The model under review builds one solid part; all positions refer to its coordinate system, in mm. Coordinates: 2 decimals unless noted, no trailing zeros. Write each question's results on one line, items separated by ' | '.
from build123d import *

# Parameters (mm, degrees)
EXTRUDE1_DEPTH = 406.4


with BuildPart() as part:
    # Sketch1 → Extrude1 (new body)
    with BuildSketch(Plane.XY):
        with BuildLine():
            Line((8.3439, -10.4902), (6.225100202, -10.4902))
            ThreePointArc((6.225100202, -10.4902), (5.286438597, -9.863006367), (5.506679712, -8.75577951))
            Line((5.506679712, -8.75577951), (8.81535611, -5.447103113))
            ThreePointArc((8.81535611, -5.447103113), (9.845400242, -4.758849627), (11.06042014, -4.517167143))
            Line((11.06042014, -4.517167143), (14.33957986, -4.517167143))
            ThreePointArc((14.33957986, -4.517167143), (15.554599758, -4.758849627), (16.58464389, -5.447103113))
            Line((16.58464389, -5.447103113), (19.893320288, -8.75577951))
            ThreePointArc((19.893320288, -8.75577951), (20.113561403, -9.863006367), (19.174899798, -10.4902))
            Line((19.174899798, -10.4902), (17.0561, -10.4902))
            ThreePointArc((17.0561, -10.4902), (15.9512, -11.5951), (17.0561, -12.7))
            Line((17.0561, -12.7), (23.2918, -12.7))
            ThreePointArc((23.2918, -12.7), (24.782522516, -12.082522516), (25.4, -10.5918))
            Line((25.4, -10.5918), (25.4, -4.3561))
            ThreePointArc((25.4, -4.3561), (24.2951, -3.2512), (23.1902, -4.3561))
            Line((23.1902, -4.3561), (23.1902, -6.474899798))
            ThreePointArc((23.1902, -6.474899798), (22.563006367, -7.413561403), (21.45577951, -7.193320288))
            Line((21.45577951, -7.193320288), (18.147103113, -3.88464389))
            ThreePointArc((18.147103113, -3.88464389), (17.458849627, -2.854599758), (17.217167143, -1.63957986))
            Line((17.217167143, -1.63957986), (17.217167143, 1.63957986))
            ThreePointArc((17.217167143, 1.63957986), (17.458849627, 2.854599758), (18.147103113, 3.88464389))
            Line((18.147103113, 3.88464389), (21.45577951, 7.193320288))
            ThreePointArc((21.45577951, 7.193320288), (22.563006367, 7.413561403), (23.1902, 6.474899798))
            Line((23.1902, 6.474899798), (23.1902, 4.3561))
            ThreePointArc((23.1902, 4.3561), (24.2951, 3.2512), (25.4, 4.3561))
            Line((25.4, 4.3561), (25.4, 10.5918))
            ThreePointArc((25.4, 10.5918), (24.782522516, 12.082522516), (23.2918, 12.7))
            Line((23.2918, 12.7), (17.0561, 12.7))
            ThreePointArc((17.0561, 12.7), (15.9512, 11.5951), (17.0561, 10.4902))
            Line((17.0561, 10.4902), (19.174899798, 10.4902))
            ThreePointArc((19.174899798, 10.4902), (20.113561403, 9.863006367), (19.893320288, 8.75577951))
            Line((19.893320288, 8.75577951), (16.58464389, 5.447103113))
            ThreePointArc((16.58464389, 5.447103113), (15.554599758, 4.758849627), (14.33957986, 4.517167143))
            Line((14.33957986, 4.517167143), (11.06042014, 4.517167143))
            ThreePointArc((11.06042014, 4.517167143), (9.845400242, 4.758849627), (8.81535611, 5.447103113))
            Line((8.81535611, 5.447103113), (5.506679712, 8.75577951))
            ThreePointArc((5.506679712, 8.75577951), (5.286438597, 9.863006367), (6.225100202, 10.4902))
            Line((6.225100202, 10.4902), (8.3439, 10.4902))
            ThreePointArc((8.3439, 10.4902), (9.4488, 11.5951), (8.3439, 12.7))
            Line((8.3439, 12.7), (-8.3439, 12.7))
            ThreePointArc((-8.3439, 12.7), (-9.4488, 11.5951), (-8.3439, 10.4902))
            Line((-8.3439, 10.4902), (-6.225100202, 10.4902))
            ThreePointArc((-6.225100202, 10.4902), (-5.286438597, 9.863006367), (-5.506679712, 8.75577951))
            Line((-5.506679712, 8.75577951), (-8.81535611, 5.447103113))
            ThreePointArc((-8.81535611, 5.447103113), (-9.845400242, 4.758849627), (-11.06042014, 4.517167143))
            Line((-11.06042014, 4.517167143), (-14.33957986, 4.517167143))
            ThreePointArc((-14.33957986, 4.517167143), (-15.554599758, 4.758849627), (-16.58464389, 5.447103113))
            Line((-16.58464389, 5.447103113), (-19.893320288, 8.75577951))
            ThreePointArc((-19.893320288, 8.75577951), (-20.113561403, 9.863006367), (-19.174899798, 10.4902))
            Line((-19.174899798, 10.4902), (-17.0561, 10.4902))
            ThreePointArc((-17.0561, 10.4902), (-15.9512, 11.5951), (-17.0561, 12.7))
            Line((-17.0561, 12.7), (-23.2918, 12.7))
            ThreePointArc((-23.2918, 12.7), (-24.782522516, 12.082522516), (-25.4, 10.5918))
            Line((-25.4, 10.5918), (-25.4, 4.3561))
            ThreePointArc((-25.4, 4.3561), (-24.2951, 3.2512), (-23.1902, 4.3561))
            Line((-23.1902, 4.3561), (-23.1902, 6.474899798))
            ThreePointArc((-23.1902, 6.474899798), (-22.563006367, 7.413561403), (-21.45577951, 7.193320288))
            Line((-21.45577951, 7.193320288), (-18.147103113, 3.88464389))
            ThreePointArc((-18.147103113, 3.88464389), (-17.458849627, 2.854599758), (-17.217167143, 1.63957986))
            Line((-17.217167143, 1.63957986), (-17.217167143, -1.63957986))
            ThreePointArc((-17.217167143, -1.63957986), (-17.458849627, -2.854599758), (-18.147103113, -3.88464389))
            Line((-18.147103113, -3.88464389), (-21.45577951, -7.193320288))
            ThreePointArc((-21.45577951, -7.193320288), (-22.563006367, -7.413561403), (-23.1902, -6.474899798))
            Line((-23.1902, -6.474899798), (-23.1902, -4.3561))
            ThreePointArc((-23.1902, -4.3561), (-24.2951, -3.2512), (-25.4, -4.3561))
            Line((-25.4, -4.3561), (-25.4, -10.5918))
            ThreePointArc((-25.4, -10.5918), (-24.782522516, -12.082522516), (-23.2918, -12.7))
            Line((-23.2918, -12.7), (-17.0561, -12.7))
            ThreePointArc((-17.0561, -12.7), (-15.9512, -11.5951), (-17.0561, -10.4902))
            Line((-17.0561, -10.4902), (-19.174899798, -10.4902))
            ThreePointArc((-19.174899798, -10.4902), (-20.113561403, -9.863006367), (-19.893320288, -8.75577951))
            Line((-19.893320288, -8.75577951), (-16.58464389, -5.447103113))
            ThreePointArc((-16.58464389, -5.447103113), (-15.554599758, -4.758849627), (-14.33957986, -4.517167143))
            Line((-14.33957986, -4.517167143), (-11.06042014, -4.517167143))
            ThreePointArc((-11.06042014, -4.517167143), (-9.845400242, -4.758849627), (-8.81535611, -5.447103113))
            Line((-8.81535611, -5.447103113), (-5.506679712, -8.75577951))
            ThreePointArc((-5.506679712, -8.75577951), (-5.286438597, -9.863006367), (-6.225100202, -10.4902))
            Line((-6.225100202, -10.4902), (-8.3439, -10.4902))
            ThreePointArc((-8.3439, -10.4902), (-9.4488, -11.5951), (-8.3439, -12.7))
            Line((-8.3439, -12.7), (8.3439, -12.7))
            ThreePointArc((8.3439, -12.7), (9.4488, -11.5951), (8.3439, -10.4902))
        make_face()
        with BuildLine():
            Line((-14.040533428, -2.231856263), (-14.669151357, -2.860474191))
            ThreePointArc((-14.669151357, -2.860474191), (-15.618583239, -2.918583239), (-15.560474191, -1.969151357))
            Line((-15.560474191, -1.969151357), (-14.931856263, -1.340533428))
            ThreePointArc((-14.931856263, -1.340533428), (-15.3035, 0), (-14.931856263, 1.340533428))
            Line((-14.931856263, 1.340533428), (-15.560474191, 1.969151357))
            ThreePointArc((-15.560474191, 1.969151357), (-15.618583239, 2.918583239), (-14.669151357, 2.860474191))
            Line((-14.669151357, 2.860474191), (-14.040533428, 2.231856263))
            ThreePointArc((-14.040533428, 2.231856263), (-12.7, 2.6035), (-11.359466572, 2.231856263))
            Line((-11.359466572, 2.231856263), (-10.730848643, 2.860474191))
            ThreePointArc((-10.730848643, 2.860474191), (-9.781416761, 2.918583239), (-9.839525809, 1.969151357))
            Line((-9.839525809, 1.969151357), (-10.468143737, 1.340533428))
            ThreePointArc((-10.468143737, 1.340533428), (-10.0965, 0), (-10.468143737, -1.340533428))
            Line((-10.468143737, -1.340533428), (-9.839525809, -1.969151357))
            ThreePointArc((-9.839525809, -1.969151357), (-9.781416761, -2.918583239), (-10.730848643, -2.860474191))
            Line((-10.730848643, -2.860474191), (-11.359466572, -2.231856263))
            ThreePointArc((-11.359466572, -2.231856263), (-12.7, -2.6035), (-14.040533428, -2.231856263))
        make_face(mode=Mode.SUBTRACT)
        with BuildLine():
            Line((14.669151357, -2.860474191), (14.040533428, -2.231856263))
            ThreePointArc((14.040533428, -2.231856263), (12.7, -2.6035), (11.359466572, -2.231856263))
            Line((11.359466572, -2.231856263), (10.730848643, -2.860474191))
            ThreePointArc((10.730848643, -2.860474191), (9.781416761, -2.918583239), (9.839525809, -1.969151357))
            Line((9.839525809, -1.969151357), (10.468143737, -1.340533428))
            ThreePointArc((10.468143737, -1.340533428), (10.0965, 0), (10.468143737, 1.340533428))
            Line((10.468143737, 1.340533428), (9.839525809, 1.969151357))
            ThreePointArc((9.839525809, 1.969151357), (9.781416761, 2.918583239), (10.730848643, 2.860474191))
            Line((10.730848643, 2.860474191), (11.359466572, 2.231856263))
            ThreePointArc((11.359466572, 2.231856263), (12.7, 2.6035), (14.040533428, 2.231856263))
            Line((14.040533428, 2.231856263), (14.669151357, 2.860474191))
            ThreePointArc((14.669151357, 2.860474191), (15.618583239, 2.918583239), (15.560474191, 1.969151357))
            Line((15.560474191, 1.969151357), (14.931856263, 1.340533428))
            ThreePointArc((14.931856263, 1.340533428), (15.3035, 0), (14.931856263, -1.340533428))
            Line((14.931856263, -1.340533428), (15.560474191, -1.969151357))
            ThreePointArc((15.560474191, -1.969151357), (15.618583239, -2.918583239), (14.669151357, -2.860474191))
        make_face(mode=Mode.SUBTRACT)
        with BuildLine():
            Line((-0.45223726, 10.033), (0.45223726, 10.033))
            ThreePointArc((0.45223726, 10.033), (1.054887129, 9.913125488), (1.565789019, 9.571751759))
            Line((1.565789019, 9.571751759), (7.252896887, 3.88464389))
            ThreePointArc((7.252896887, 3.88464389), (7.941150373, 2.854599758), (8.182832857, 1.63957986))
            Line((8.182832857, 1.63957986), (8.182832857, -1.63957986))
            ThreePointArc((8.182832857, -1.63957986), (7.941150373, -2.854599758), (7.252896887, -3.88464389))
            Line((7.252896887, -3.88464389), (1.565789019, -9.571751759))
            ThreePointArc((1.565789019, -9.571751759), (1.054887129, -9.913125488), (0.45223726, -10.033))
            Line((0.45223726, -10.033), (-0.45223726, -10.033))
            ThreePointArc((-0.45223726, -10.033), (-1.054887129, -9.913125488), (-1.565789019, -9.571751759))
            Line((-1.565789019, -9.571751759), (-7.252896887, -3.88464389))
            ThreePointArc((-7.252896887, -3.88464389), (-7.941150373, -2.854599758), (-8.182832857, -1.63957986))
            Line((-8.182832857, -1.63957986), (-8.182832857, 1.63957986))
            ThreePointArc((-8.182832857, 1.63957986), (-7.941150373, 2.854599758), (-7.252896887, 3.88464389))
            Line((-7.252896887, 3.88464389), (-1.565789019, 9.571751759))
            ThreePointArc((-1.565789019, 9.571751759), (-1.054887129, 9.913125488), (-0.45223726, 10.033))
        make_face(mode=Mode.SUBTRACT)
    extrude(amount=-EXTRUDE1_DEPTH)


solid = part.part
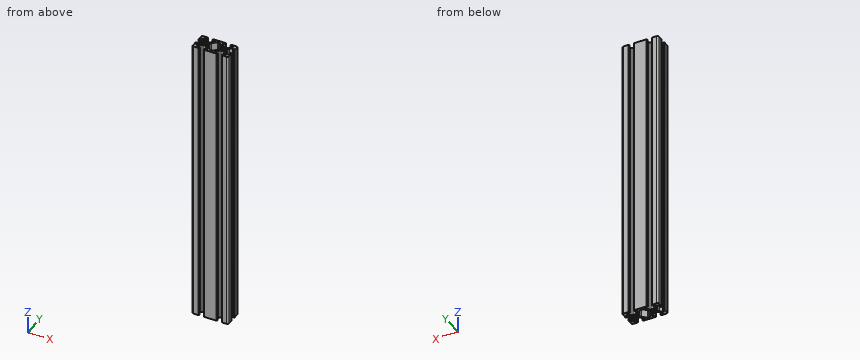
1) For pin 1 (2.5 mm diameter, centred on y = 0.5, z = -157, fed in from +X); pin 2 (3 mm diameter, centred on x = 13.5, z = -200, fed in from +Y); pin 3 (3.5 mm diameter, centred on y = -0.5, z = -298.5, fed in from -X), all flat-tipped, find the tip position at first contact; note any pin that passes through.
Solutions:
pin 1: x = 17.22 | pin 2: y = 4.59 | pin 3: x = -17.28
2) To check wall thickness, follow line 1 along X through (y, z) = (0.5, -30.5); line 2 along X through (y, z) = (-9.5, -151); line 3 along X through (y, z) = (-6.25, -200.5). State the ranges of each line that lie inside material, in increasing order.
Solutions:
line 1: -17.22 to -15.26, -10.14 to -8.18, 8.18 to 10.14, 15.26 to 17.22 | line 2: -25.4 to -20.19, -5.21 to -1.64, 1.64 to 5.21, 20.19 to 25.4 | line 3: -25.4 to -23.19, -20.51 to -17.39, -8.01 to -4.89, 4.89 to 8.01, 17.39 to 20.51, 23.19 to 25.4
3) Take a section at A-A on z = -206.5. Count the separate pieces of the cut face and the enclosed holes in it, plus the area to 3 significant figures.
Solutions:
separate pieces: 1 | enclosed holes: 3 | area: 502 mm2
